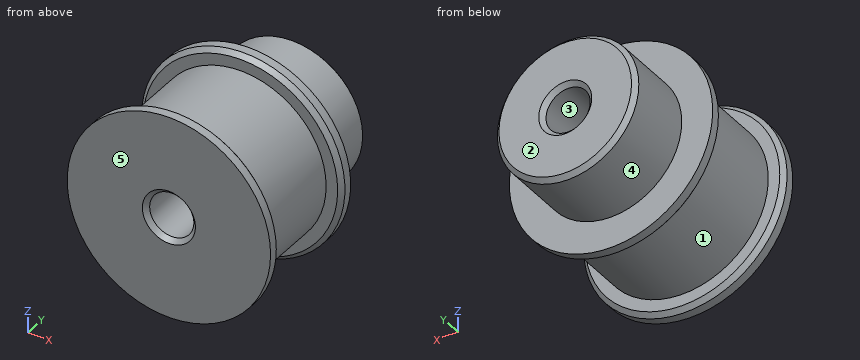
from build123d import *

# Parameters (mm, degrees)
F0_R     = 9.7
F1_DEPTH = 5.5
F2_R     = 11.5
F3_DEPTH = 1.5
F4_R     = 11.5
F5_DEPTH = 1.5
F6_R     = 8
F7_DEPTH = 8
F8_R     = 2.5
F9_DEPTH = 22.001
F10_SIZE = 0.5


with BuildPart() as f1:
    # F0 (on Front) → F1 (new body, symmetric)
    with BuildSketch(Plane.XZ):
        Circle(F0_R)
    extrude(amount=F1_DEPTH, both=True)

    # F2 (on face) → F3 (join)
    with BuildSketch(Plane.XZ.offset(5.5)):
        Circle(F2_R)
    extrude(amount=F3_DEPTH)

    # F4 (on face) → F5 (join)
    with BuildSketch(Plane(origin=(0, 5.5, 0), x_dir=(-1, 0, 0), z_dir=(0, 1, 0))):
        Circle(F4_R)
    extrude(amount=F5_DEPTH)

    # F6 (on face) → F7 (join)
    with BuildSketch(Plane(origin=(0, 7, 0), x_dir=(-1, 0, 0), z_dir=(0, 1, 0))):
        Circle(F6_R)
    extrude(amount=F7_DEPTH)

    # F8 (on face) → F9 (cut, through all)
    with BuildSketch(Plane(origin=(0, 15, 0), x_dir=(-1, 0, 0), z_dir=(0, 1, 0))):
        Circle(F8_R)
    extrude(amount=-F9_DEPTH, mode=Mode.SUBTRACT)

    # F10
    f10_edges = [f1.edges().sort_by_distance(p)[0] for p in [
        (2.5, -7, 0),
        (2.5, 15, 0),
        (-11.5, -5.5, 0),
        (11.5, 5.5, 0),
        (8, 15, 0),
    ]]
    chamfer(f10_edges, length=F10_SIZE)


solid = f1.part
Geometry: final body of the model. Coordinates: model frame, mm. Face numbers are marked on the shaded views. A direction names the side the tool comes from. Coordinates: 2 decimals unless noted, no trailing zeros. Write each loop counter-clockwise with the first axis right and the second up, starting at its lowest first coordinate (ties: lowest second). Pieces come first, ordered by that corner, then holes. Notation, with made-up numbers: (21, 48) - (63, 48) arc R5 ccw to (63, 56) - close; hole circle Ø5 at (88.25, -32). An arc over 180 degrees is marked (long way). Return JSON: item names as keys, results as strings.
Item 1: Reachability of the marked faces 4 and 5 from +Z, -Z, +X, -X, +Y, -Y: full face, straight path, thin tool, end or side. Return the list, or none.
Completed:
{"face 4": "+Y", "face 5": "+Z, -Z, +X, -X, -Y"}
Item 2: Pin query (flat end, axial travel): pin 1 Ø3 at (y, z) = (10.5, 8.5) entering from +X; pin 2 Ø1 at (x, y) = (-4.5, 0) entering from -Z; pin 3 Ø3 at (y, z) = (-2, 2.5) entering from -X. Return the tip coordinate at first contact, or that it passes through.
Completed:
{"pin 1": "stops at x = 3.87", "pin 2": "stops at z = -8.84", "pin 3": "stops at x = -9.65"}
Item 3: Section query C-C (y = 12). Output: boundary loops of the cut face in (x, z).
Completed:
{"outline": "circle Ø16 at (0, 0); hole circle Ø5 at (0, 0)"}
Item 4: Line query: L1, parallel to Z at x = 0, y = 1; L2, parallel to Y at x = 7.75, z = -7.5; L3, parallel to Y at x = 8.5, z = 0.25. Output: solid intervals per line, ascending.
Completed:
{"L1": "z = -9.7 to -2.5, 2.5 to 9.7", "L2": "y = -7 to -5.5, 5.5 to 7", "L3": "y = -7 to 7"}
Item 5: Pull-direction query (Z, two-part tool) for the marked faces 1, 2 and 3; classes: +Z half, -Z half, draft (parallel to the pull), parting line (faces both ways), or undercut.
Completed:
{"face 1": "parting line", "face 2": "draft", "face 3": "undercut"}
Item 6: Section query D-D (y = -1.25). Output: boundary loops of the cut face in (x, z).
Completed:
{"outline": "circle Ø19.4 at (0, 0); hole circle Ø5 at (0, 0)"}
